Verification items for the finished model (mm, model axes). A direction names the side the tool comes from. Coordinates: 2 decimals unless noted, no trailing zeros. Loops run counter-clockwise (first coordinate to the right, second up) from the corner with the lowest first, then second, coordinate; pieces in that order, holes last. Notation, with made-up numbers: (-9, 18.5) - (22, 18.5) arc R19 cw to (22, 53.5) - close; hole circle Ø11 at (-3.5, -30). An arc over 180 degrees is marked (long way). One line per item, written item: value. Start each with the question number.
(1) Thickness scan on probe 1 along Z at (x, y) = (1, -9); probe 2 along Z at (x, y) = (19.5, 1.5); probe 3 along Y at (x, z) = (16, 5). Record the ranges inside material, lowest first. Write a range as [from, to].
(2) Section check A-A (x = 19). Record the boundary of the cut face in (y, z).
(3) Gauge pin test, flat ends, axial feed: P1, Ø1, axis at x = 6.5, z = -26.5, coming from the -Y side; P2, Ø7, axis at y = 24, z = -5, coming from the -X side; P3, Ø3, axis at x = 12, z = -17, coming from the -Y side; P4, Ø5, axis at x = -4.5, z = -8.5, coming from the -Y side. Record the tip position at first contact, or that the pin passes through.
(4) Set-up check for faces 5 (the face through (14, -15.3, -26)), 6 (the face through (10, 24, 5)), 7 (the face through (10, 0, 10.25)), 8 (the face through (14, 14.7, -26)): record each of +Z, -Z, +X, -X, +Y, -Y from which the full face is reachable in a straight line by a thin tool's end or side.
(5) Section check D-D (z = -1). Record the boundary of the cut face in (x, y).
(6) Section check B-B (y = 17). Record the boundary of the cut face in (x, z), plus the area to 3 significant figures.
(7) Section check C-C (y = 11). Record the boundary of the cut face in (x, z), plus the area to 3 significant figures.
(8) Draft check along Y on faces 1 (the face through (10, 15, -13.25)), 2 (the face through (15.132, 26.245, -5.148)), 3 (the face through (10.06, 24.93, 11.52)), 4 (the face through (10.06, -5.87, -22.65)). Enter one of: +Y half, -Y half, draft (parallel to the pull), parting line (faces both ways), or undercut.
```python
from build123d import *

# Parameters (mm, degrees)
SKETCH1_R           = 2.25
BOSS_EXTRUDE1_DEPTH = 20
SKETCH2_R           = 2.25
BOSS_EXTRUDE2_DEPTH = 10
SKETCH4_W           = 26.5
SKETCH4_H           = 2.5
CUT_EXTRUDE1_DEPTH  = 39.17921555
CHAMFER2_SIZE       = 4
CHAMFER3_SIZE       = 4
FILLET4_R           = 2
SKETCH7_W           = 10
SKETCH7_H           = 10
BOSS_EXTRUDE5_DEPTH = 20
FILLET6_R           = 2
SKETCH8_W           = 63
SKETCH8_H           = 30
BOSS_EXTRUDE6_DEPTH = 4
CHAMFER4_SIZE       = 2
FILLET7_R           = 2
SKETCH13_R          = 2.25
BOSS_EXTRUDE7_DEPTH = 0.41


with BuildPart() as part:
    # Sketch1 → Boss-Extrude1 (new body)
    with BuildSketch(Plane(origin=(0, 0, 0), x_dir=(0, 0, -1), z_dir=(1, 0, 0))):
        Polygon((10.25, -20.3), (13.25, -20.3), (13.25, 29.7), (-13.25, 29.7), (-13.25, -20.3), (-10.25, -20.3), (-10.25, 20.3), (10.25, 20.3), align=None)
        with Locations((5, 24)):
            Circle(SKETCH1_R, mode=Mode.SUBTRACT)
        with Locations((-5, 24)):
            Circle(SKETCH1_R, mode=Mode.SUBTRACT)
    extrude(amount=BOSS_EXTRUDE1_DEPTH)

    # Sketch2 → Boss-Extrude2 (add)
    with BuildSketch(Plane.ZY):
        with Locations((-5, 24)):
            Circle(SKETCH2_R)
        with Locations((5, 24)):
            Circle(SKETCH2_R)
    extrude(amount=-BOSS_EXTRUDE2_DEPTH)

    # Sketch4 → Cut-Extrude1 (cut, through all)
    with BuildSketch(Plane(origin=(20, 0, 0), x_dir=(0, 0, -1), z_dir=(1, 0, 0))):
        with Locations((0, 28.45)):
            Rectangle(SKETCH4_W, SKETCH4_H)
    extrude(amount=-CUT_EXTRUDE1_DEPTH, mode=Mode.SUBTRACT)

    # Chamfer2
    chamfer2_edges = [part.edges().sort_by_distance(p)[0] for p in [
        (10, 27.2, -13.25),
    ]]
    chamfer(chamfer2_edges, length=CHAMFER2_SIZE)

    # Chamfer3
    chamfer3_edges = [part.edges().sort_by_distance(p)[0] for p in [
        (10, 27.2, 13.25),
    ]]
    chamfer(chamfer3_edges, length=CHAMFER3_SIZE)

    # Fillet4
    fillet4_edges = [part.edges().sort_by_distance(p)[0] for p in [
        (10, 27.2, -9.25),
        (10, 27.2, 9.25),
    ]]
    fillet(fillet4_edges, radius=FILLET4_R)

    # Sketch7 → Boss-Extrude5 (add)
    with BuildSketch(Plane(origin=(20, 0, 0), x_dir=(0, 0, -1), z_dir=(1, 0, 0))):
        with Locations((18.25, -0.3)):
            Rectangle(SKETCH7_W, SKETCH7_H)
    extrude(amount=-BOSS_EXTRUDE5_DEPTH)

    # Fillet6
    fillet6_edges = [part.edges().sort_by_distance(p)[0] for p in [
        (10, -5.3, -13.25),
        (10, 4.7, -13.25),
    ]]
    fillet(fillet6_edges, radius=FILLET6_R)

    # Sketch8 → Boss-Extrude6 (add)
    with BuildSketch(Plane(origin=(0, 0, -23.25), x_dir=(-1, 0, 0), z_dir=(0, 0, -1))):
        with Locations((-13.9, -0.3)):
            Rectangle(SKETCH8_W, SKETCH8_H)
    extrude(amount=BOSS_EXTRUDE6_DEPTH)

    # Chamfer4
    chamfer4_edges = [part.edges().sort_by_distance(p)[0] for p in [
        (45.4, -0.3, -23.25),
        (13.9, -15.3, -23.25),
        (-17.6, -0.3, -23.25),
        (13.9, 14.7, -23.25),
    ]]
    chamfer(chamfer4_edges, length=CHAMFER4_SIZE)

    # Fillet7
    fillet7_edges = [part.edges().sort_by_distance(p)[0] for p in [
        (10, 4.7, -23.25),
        (10, -5.3, -23.25),
    ]]
    fillet(fillet7_edges, radius=FILLET7_R)

    # Sketch13 → Boss-Extrude7 (add)
    with BuildSketch(Plane(origin=(20, 0, 0), x_dir=(0, 0, -1), z_dir=(1, 0, 0))):
        with BuildLine():
            Line((13.25, 23.2), (9.835786438, 26.614213562))
            ThreePointArc((9.835786438, 26.614213562), (9.18693974, 27.047759065), (8.421572875, 27.2))
            Line((8.421572875, 27.2), (-8.421572875, 27.2))
            ThreePointArc((-8.421572875, 27.2), (-9.18693974, 27.047759065), (-9.835786438, 26.614213562))
            Line((-9.835786438, 26.614213562), (-13.25, 23.2))
            Line((-13.25, 23.2), (-13.25, -20.3))
            Line((-13.25, -20.3), (-10.25, -20.3))
            Line((-10.25, -20.3), (-10.25, 20.3))
            Line((-10.25, 20.3), (10.25, 20.3))
            Line((10.25, 20.3), (10.25, -20.3))
            Line((10.25, -20.3), (13.25, -20.3))
            Line((13.25, -20.3), (13.25, -7.3))
            ThreePointArc((13.25, -7.3), (13.835786438, -5.885786438), (15.25, -5.3))
            Line((15.25, -5.3), (21.25, -5.3))
            ThreePointArc((21.25, -5.3), (22.664213562, -5.885786438), (23.25, -7.3))
            Line((23.25, -7.3), (23.25, 6.7))
            ThreePointArc((23.25, 6.7), (22.664213562, 5.285786438), (21.25, 4.7))
            Line((21.25, 4.7), (15.25, 4.7))
            ThreePointArc((15.25, 4.7), (13.835786438, 5.285786438), (13.25, 6.7))
            Line((13.25, 6.7), (13.25, 23.2))
        make_face()
        with Locations(Location((5, 24, 0), (0, 0, 180))):
            Circle(SKETCH13_R, mode=Mode.SUBTRACT)
        with Locations(Location((-5, 24, 0), (0, 0, 180))):
            Circle(SKETCH13_R, mode=Mode.SUBTRACT)
    extrude(amount=BOSS_EXTRUDE7_DEPTH)


solid = part.part
```
Responses:
1. probe 1: z = [-27.25, -23.25], [-13.25, -10.25], [10.25, 13.25]
1. probe 2: z = [-27.25, -10.25], [10.25, 13.25]
1. probe 3: y = [20.3, 21.75], [26.25, 27.2]
2. outline: (-20.3, -13.25) - (-7.3, -13.25) arc R2 cw to (-5.3, -15.25) - (-5.3, -21.25) arc R2 cw to (-7.3, -23.25) - (-13.3, -23.25) - (-15.3, -25.25) - (-15.3, -27.25) - (14.7, -27.25) - (14.7, -25.25) - (12.7, -23.25) - (6.7, -23.25) arc R2 cw to (4.7, -21.25) - (4.7, -15.25) arc R2 cw to (6.7, -13.25) - (23.2, -13.25) - (26.61, -9.84) arc R2 ccw to (27.2, -8.42) - (27.2, 8.42) arc R2 ccw to (26.61, 9.84) - (23.2, 13.25) - (-20.3, 13.25) - (-20.3, 10.25) - (20.3, 10.25) - (20.3, -10.25) - (-20.3, -10.25) - close; hole circle Ø4.5 at (24, -5); hole circle Ø4.5 at (24, 5)
3. P1: stops at y = -15.3
3. P2: stops at x = 0
3. P3: stops at y = -5.3
3. P4: passes through
4. face 5: -Z, +X, -X, -Y
4. face 6: +X
4. face 7: +X, -X, -Y
4. face 8: -Z, +X, -X, +Y
5. outline: (0, 20.3) - (20.41, 20.3) - (20.41, 27.2) - (0, 27.2) - close
6. outline: (0, -13.25) - (20.41, -13.25) - (20.41, -10.25) - (0, -10.25) - close; (0, 10.25) - (20.41, 10.25) - (20.41, 13.25) - (0, 13.25) - close
6. area: 122 mm²
7. outline: (-17.6, -27.25) - (45.4, -27.25) - (45.4, -25.25) - (43.4, -23.25) - (-15.6, -23.25) - (-17.6, -25.25) - close; (0, -13.25) - (20.41, -13.25) - (20.41, -10.25) - (0, -10.25) - close; (0, 10.25) - (20.41, 10.25) - (20.41, 13.25) - (0, 13.25) - close
7. area: 370 mm²
8. face 1: draft
8. face 2: undercut
8. face 3: +Y half
8. face 4: -Y half
